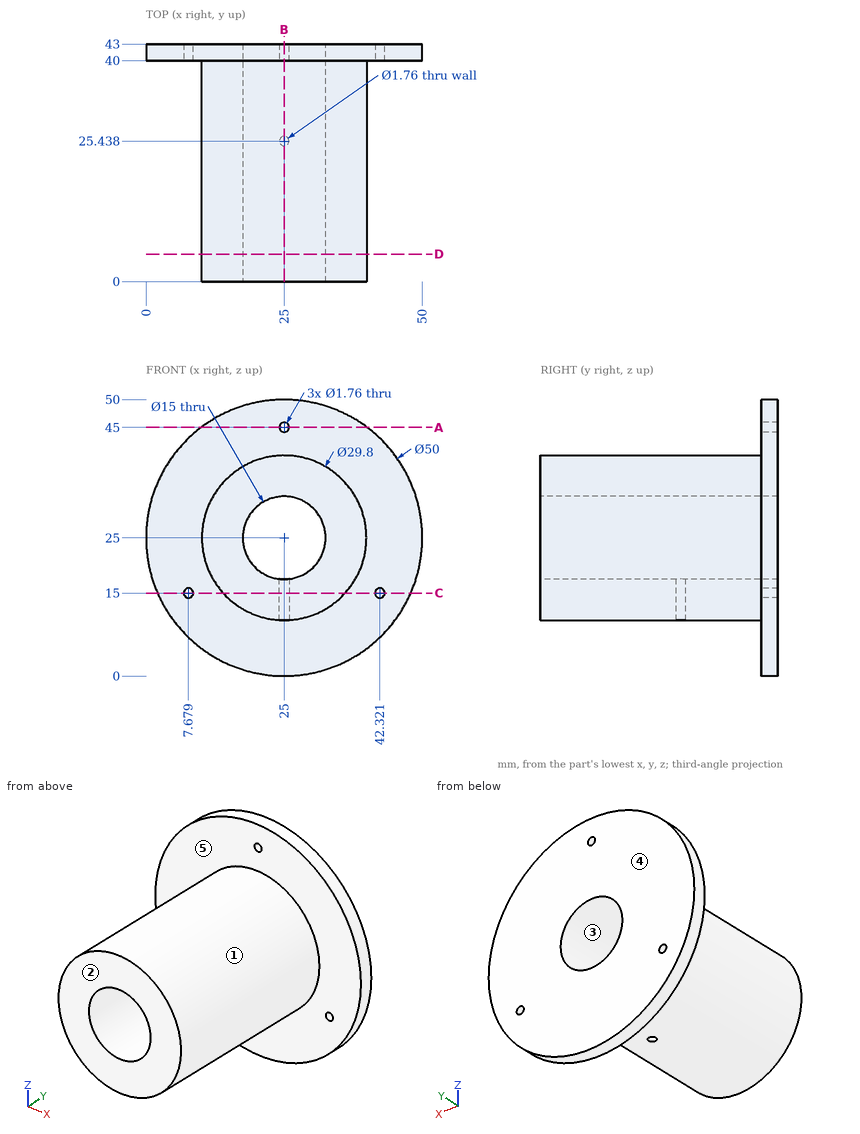
Here's the drawing with two shaded views (mm, measured from the low corner). I have some questions. A direction names the side the tool comes from. Round coordinates to 2 decimals unless told otherwise and drop trailing zeros. Loops run counter-clockwise (first coordinate to the right, second up) from the corner with the lowest first, then second, coordinate; pieces in that order, holes last.
Item 1: Suppose I cut it at D-D, the plane y = 5. Write out the boundary of the cut face in (x, z).
Item 2: Suppose I cut it at C-C, the plane z = 15. Write out the boundary of the cut face in (x, y) (1 decimal), then the cut area to 3 significant figures.
Item 3: Will these pins go through, and if not, where does the flat tip stop? pin 1 Ø6 at (y, z) = (30.5, 18) entering from +X; pin 2 Ø1.4 at (x, z) = (7.68, 15) entering from +Y; pin 3 Ø6 at (x, y) = (38, 17.5) entering from +Z (1 decimal); pin 4 Ø10 at (x, y) = (42.5, 5) entering from -Z.
Item 4: If we mould it in two halves opening along X, with no side actions, what happens to the marked faces 1, 2 and 3? For each: +X half, -X half, draft (parallel to the pull), parting line (faces both ways), or undercut.
Item 5: Which directions (+Z, -Z, +X, -X, +Y, -Y) give clear straight access to the entire face, cutting with the end or side of a thin tool? Please do the marked faces 4 and 5.
Item 6: Please list where these lines run through material, in increasing order: L1, parallel to Z at x = 25, y = 41.95; L2, parallel to Z at x = 25, y = 11.5; L3, parallel to X at y = 13, z = 31 (1 decimal).
Item 7: Suppose I cut it at B-B, the plane x = 25. Write out the boundary of the cut face in (y, z).
Item 8: Suppose I cut it at A-A, the plane z = 45. Write out the boundary of the cut face in (x, y).
Reported:
1. outline: circle Ø29.8 at (25, 25); hole circle Ø15 at (25, 25)
2. outline: (2.1, 40) - (6.8, 40) - (6.8, 43) - (2.1, 43) - close; (8.6, 40) - (14, 40) - (14, 0) - (36, 0) - (36, 40) - (41.4, 40) - (41.4, 43) - (8.6, 43) - close; (43.2, 40) - (47.9, 40) - (47.9, 43) - (43.2, 43) - close; hole circle Ø1.8 at (25, 25.4)
2. area: 1,010 mm2
3. pin 1: stops at x = 39.35
3. pin 2: passes through
3. pin 3: stops at z = 36
3. pin 4: stops at z = 16.89
4. face 1: parting line
4. face 2: draft
4. face 3: undercut
5. face 4: +Z, -Z, +X, -X, +Y
5. face 5: -Y
6. L1: z = 0 to 17.5, 32.5 to 44.12, 45.88 to 50
6. L2: z = 10.1 to 17.5, 32.5 to 39.9
6. L3: x = 11.4 to 20.5, 29.5 to 38.6
7. outline: (0, 10.1) - (24.56, 10.1) - (24.56, 17.5) - (0, 17.5) - close; (0, 32.5) - (43, 32.5) - (43, 44.12) - (40, 44.12) - (40, 39.9) - (0, 39.9) - close; (26.32, 10.1) - (40, 10.1) - (40, 0) - (43, 0) - (43, 17.5) - (26.32, 17.5) - close; (40, 45.88) - (43, 45.88) - (43, 50) - (40, 50) - close
8. outline: (10, 40) - (24.12, 40) - (24.12, 43) - (10, 43) - close; (25.88, 40) - (40, 40) - (40, 43) - (25.88, 43) - close
